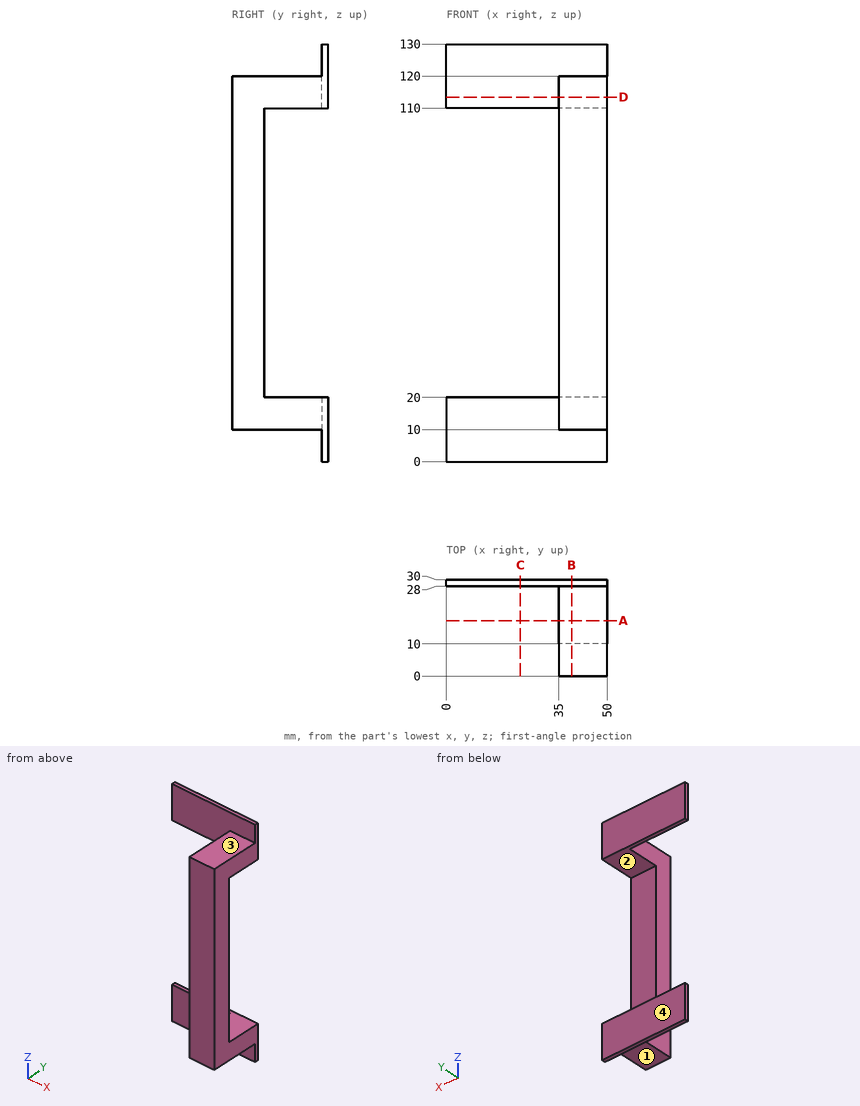
Study the drawing (mm; zero at the part's minimum x, y, z) and answer. A direction names the side the tool comes from. Give positions to 0.01 mm unless a question says otherwise; leave off trailing zeros. Loops run counter-clockwise (first coordinate to the right, second up) from the corner with the lowest first, then second, coordinate; pieces in that order, holes last. Notation, with made-up numbers: M -15,-15.75 L 19,-15.75 A36 ccw 19,23.25 Z; hole C 66,-22 d2. An arc over 180 degrees is marked long. One line per item, written item: value. Start each with the question number.
1. Find section C-C (x = 23). Give the vertices of the cut face in (y, z).
2. Find section B-B (x = 39). Give the vertices of the cut face in (y, z).
3. Find section D-D (z = 113.5). Give the vertices of the cut face in (x, y), and give its area (3 significant figures).
4. Find section A-A (y = 17.25). Give the vertices of the cut face in (x, z), and give its area (3 significant figures).
5. Each of these flat-tipped pins is pushed along its axis until it touches: P1, Ø3, axis at y = 15.5, z = 110, coming from the -X side; P2, Ø3, axis at x = 34.5, z = 47, coming from the -Y side; P3, Ø22, axis at x = 22.5, z = 12, coming from the -Y side; P4, Ø16.5, axis at x = 39, y = 17, coming from the +Z side. Where does it stop, or does it pass through?
6. Which of the six approach directions +Z, -Z, +X, -X, +Y, -Y give full straight-line access (tool end or side, diameter ignored) to the marked faces 1, 2, 3 and 4?
7. Find the intervals of material crossed by probe 1 along Z at (x, y) = (46, 14.5); probe 2 along Y at (x, z) = (44.5, 46); probe 3 along X at (y, z) = (22, 18), in increasing order.
Reported:
1. outline: M 28,0 L 30,0 L 30,20 L 28,20 Z; M 28,110 L 30,110 L 30,130 L 28,130 Z
2. outline: M 0,10 L 28,10 L 28,0 L 30,0 L 30,20 L 10,20 L 10,110 L 30,110 L 30,130 L 28,130 L 28,120 L 0,120 Z
3. outline: M 0,28 L 35,28 L 35,0 L 50,0 L 50,30 L 0,30 Z
3. area: 520 mm²
4. outline: M 35,10 L 50,10 L 50,20 L 35,20 Z; M 35,110 L 50,110 L 50,120 L 35,120 Z
4. area: 300 mm²
5. P1: stops at x = 35
5. P2: stops at y = 0
5. P3: stops at y = 28
5. P4: stops at z = 120
6. face 1: -Z, +X, -X, -Y
6. face 2: +X, -X, +Y
6. face 3: +Z, +X, -X, -Y
6. face 4: +Z, -Z, +X, -X, +Y
7. probe 1: z = 10 to 20, 110 to 120
7. probe 2: y = 0 to 10
7. probe 3: x = 35 to 50
